Can you work these out from the model? Positions are in its coordinate system, mm. A direction names the side the tool comes from. Round coordinates to 2 decimals unless told otherwise and drop trailing zeros. Loops run counter-clockwise (first coordinate to the right, second up) from the corner with the lowest first, then second, coordinate; pieces in that order, holes last. Notation, with made-up numbers: (-29, -33.5) -> (26, -33.5) arc R11 ccw to (26, -23.5) -> close; hole circle Ø3 at (7, 27). An arc over 180 degrees is marked (long way). Use a Markdown table: item, result.
from build123d import *

# Parameters (mm, degrees)
SKETCH_1_R          = 6
EXTRUDE_1_DEPTH     = 182
SKETCH_2_R          = 1.5
CUT_EXTRUDE_1_DEPTH = 8.8
SKETCH_7_R          = 1.5
CUT_EXTRUDE_2_DEPTH = 8.8


with BuildPart() as part:
    # ｽｹｯﾁ1 → ﾎﾞｽ - 押し出し1 (new body)
    with BuildSketch(Plane.XY):
        Circle(SKETCH_1_R)
    extrude(amount=EXTRUDE_1_DEPTH)

    # ｽｹｯﾁ2 → ｶｯﾄ - 押し出し1 (cut)
    with BuildSketch(Plane.XY.offset(182)):
        Circle(SKETCH_2_R)
    extrude(amount=-CUT_EXTRUDE_1_DEPTH, mode=Mode.SUBTRACT)

    # ｽｹｯﾁ7 → ｶｯﾄ - 押し出し2 (cut)
    with BuildSketch(Plane(origin=(0, 0, 0), x_dir=(-1, 0, 0), z_dir=(0, 0, -1))):
        Circle(SKETCH_7_R)
    extrude(amount=-CUT_EXTRUDE_2_DEPTH, mode=Mode.SUBTRACT)


solid = part.part
1. I want a section at A-A (x = 0). Please give me the cut outline in (y, z).
Answer sheet:
| item | result |
|---|---|
| outline | (-6, 0) -> (-1.5, 0) -> (-1.5, 8.8) -> (1.5, 8.8) -> (1.5, 0) -> (6, 0) -> (6, 182) -> (1.5, 182) -> (1.5, 173.2) -> (-1.5, 173.2) -> (-1.5, 182) -> (-6, 182) -> close |
2. If we mould it in two halves opening along X, with no side actions, what happens to faces 4 (the flat face through (0, 0, 173.2)), 5 (the flat face through (1.2, -1.2, 182)), 6 (the cylindrical face through (-6, 0, 90))? For each: +X half, -X half, draft (parallel to the pull), parting line (faces both ways), or undercut.
Answer sheet:
| item | result |
|---|---|
| face 4 | undercut |
| face 5 | draft |
| face 6 | parting line |
3. I need wall thicknesses on line 1 (Y direction, x = 0, z = 179.25); line 2 (Y direction, x = -0.25, z = 121). Which ranges of each line are inside material? Lowest first, please.
Answer sheet:
| item | result |
|---|---|
| line 1 | y = -6 to -1.5, 1.5 to 6 |
| line 2 | y = -5.99 to 5.99 |
4. Which directions (+Z, -Z, +X, -X, +Y, -Y) give clear straight access to the entire face, cutting with the end or side of a thin tool? Please do faces 1 (the flat face through (1.2, -1.2, 0)), 2 (the cylindrical face through (1.5, 0.07, 4.34)), 3 (the cylindrical face through (-1.5, 0.07, 177.66)).
Answer sheet:
| item | result |
|---|---|
| face 1 | -Z, +X, -X, +Y, -Y |
| face 2 | -Z |
| face 3 | +Z |
5. I want a section at C-C (z = 27). Please give me the cut outline in (x, y).
Answer sheet:
| item | result |
|---|---|
| outline | circle Ø12 at (0, 0) |
6. Will these pins go through, and if not, where does the flat tip stop? pin 1 Ø3 at (y, z) = (-2.5, 61.5) entering from -X; pin 2 Ø3 at (y, z) = (-4, 142.5) entering from +X; pin 3 Ø1.5 at (x, z) = (4, 112) entering from +Y.
Answer sheet:
| item | result |
|---|---|
| pin 1 | stops at x = -5.92 |
| pin 2 | stops at x = 5.45 |
| pin 3 | stops at y = 5.04 |
